```python
from build123d import *

# Parameters (mm, degrees)
BOSS_EXTRU_1_DEPTH      = 3
ESQUISSE2_R             = 1.25
ENL_V_MAT_EXTRU_1_DEPTH = 8
ESQUISSE3_W             = 6
ESQUISSE3_H             = 5
BOSS_EXTRU_2_DEPTH      = 5
ENL_V_MAT_EXTRU_3_DEPTH = 7
CONG_4_R                = 0.5
CONG_5_R                = 1
ENL_V_MAT_EXTRU_5_DEPTH = 7


with BuildPart() as part:
    # Esquisse1 → Boss.-Extru.1 (new body, symmetric)
    with BuildSketch(Plane.XY):
        Polygon((-6, 0), (-2.4, 0), (-2.4, -2), (2.4, -2), (2.4, 0), (6, 0), (6, 5), (-6, 5), align=None)
    extrude(amount=BOSS_EXTRU_1_DEPTH, both=True)

    # Esquisse2 → Enlèv. mat.-Extru.1 (cut, through all)
    with BuildSketch(Plane(origin=(0, 5, 0), x_dir=(1, 0, 0), z_dir=(0, 1, 0))):
        Circle(ESQUISSE2_R)
    extrude(amount=-ENL_V_MAT_EXTRU_1_DEPTH, mode=Mode.SUBTRACT)

    # Esquisse3 → Boss.-Extru.2 (add)
    with BuildSketch(Plane.ZY.offset(6)):
        with Locations((0, 2.5)):
            Rectangle(ESQUISSE3_W, ESQUISSE3_H)
    extrude(amount=BOSS_EXTRU_2_DEPTH)

    # Esquisse7 → Enlèv. mat.-Extru.3 (cut, through all)
    with BuildSketch(Plane.XY.offset(3)):
        Polygon((-11, 5), (-9.556624327, 2.5), (-11, 0), align=None)
    extrude(amount=-ENL_V_MAT_EXTRU_3_DEPTH, mode=Mode.SUBTRACT)

    # Congé4
    cong_4_edges = [part.edges().sort_by_distance(p)[0] for p in [
        (6, 0, 0),
        (2.4, -2, 0),
        (-2.4, -2, 0),
        (6, 5, 0),
        (-11, 0, 0),
        (-11, 5, 0),
    ]]
    fillet(cong_4_edges, radius=CONG_4_R)

    # Congé5
    cong_5_edges = [part.edges().sort_by_distance(p)[0] for p in [
        (-9.556624327, 2.5, 0),
    ]]
    fillet(cong_5_edges, radius=CONG_5_R)

    # Esquisse12 → Enlèv. mat.-Extru.5 (cut, through all)
    with BuildSketch(Plane(origin=(0, 0, -3), x_dir=(-1, 0, 0), z_dir=(0, 0, -1))):
        with BuildLine():
            Line((-4.279385242, 0), (-2.4, -0.684040287))
            ThreePointArc((-2.4, -0.684040287), (-2.997672477, 0.597672477), (-4.279385242, 0))
        make_face()
        with BuildLine():
            Line((4.279385242, 0), (2.4, -0.684040287))
            ThreePointArc((2.4, -0.684040287), (2.997672477, 0.597672477), (4.279385242, 0))
        make_face()
    extrude(amount=-ENL_V_MAT_EXTRU_5_DEPTH, mode=Mode.SUBTRACT)


solid = part.part
```
The listing builds one solid part. Answer for the finished solid, in the listing's coordinates (mm). A direction names the side the tool comes from. Coordinates: 2 decimals unless noted, no trailing zeros. Loops run counter-clockwise (first coordinate to the right, second up) from the corner with the lowest first, then second, coordinate; pieces in that order, holes last. Notation, with made-up numbers: (68, 61) - (123, 61) arc R9 cw to (123, 70) - close; hole circle Ø7 at (68.5, 83). An arc over 180 degrees is marked (long way). Write item = value, one per line.
1) Section B-B (x = 0) is taken. Determine the outline of the cut face in (y, z), plus the area to 3 significant figures.
Responses:
outline = (-2, -3) - (5, -3) - (5, -1.25) - (-2, -1.25) - close; (-2, 1.25) - (5, 1.25) - (5, 3) - (-2, 3) - close
area = 24.5 mm^2
2) Each of these flat-tipped pins is pushed along its axis until it touches: P1, Ø0.9, axis at y = -1, z = -1, coming from the -X side; P2, Ø0.9, axis at y = -1, z = -1.5, coming from the +X side; P3, Ø3, axis at x = -3.5, z = -1, coming from the -Y side. Where does it stop, or does it pass through?
Responses:
P1 = -2.4
P2 = 2.4
P3 = -1.99
3) Find the intervals of material crossed by line 1 along X through (y, z) = (0.5, 0.5); line 2 along X through (y, z) = (1.5, 0); line 3 along Z through (x, y) = (0, 2), in increasing order.
Responses:
line_1 = -10.63 to -3.88, -2.8 to -1.15, 1.15 to 2.8, 3.88 to 6
line_2 = -10.13 to -1.25, 1.25 to 6
line_3 = -3 to -1.25, 1.25 to 3
4) Section C-C (y = 1.5) is taken. Determine the outline of the cut face in (x, z), plus the area to 3 significant figures.
Responses:
outline = (-10.13, -3) - (6, -3) - (6, 3) - (-10.13, 3) - close; hole circle Ø2.5 at (0, 0)
area = 91.9 mm^2
5) Section D-D (z = -1.75) is taken. Determine the outline of the cut face in (x, y).
Responses:
outline = (-10.57, 0.75) arc R0.5 ccw to (-10.13, 0) - (-4.28, 0) arc R1 cw to (-2.4, -0.68) - (-2.4, -1.5) arc R0.5 ccw to (-1.9, -2) - (1.9, -2) arc R0.5 ccw to (2.4, -1.5) - (2.4, -0.68) arc R1 cw to (4.28, 0) - (5.5, 0) arc R0.5 ccw to (6, 0.5) - (6, 4.5) arc R0.5 ccw to (5.5, 5) - (-10.13, 5) arc R0.5 ccw to (-10.57, 4.25) - (-9.85, 3) arc R1 cw to (-9.85, 2) - close
6) Which of the six approach directions +Z, -Z, +X, -X, +Y, -Y give full straight-line access (tool end or side, diameter ignored) to faces 4 (the face through (-2.4, -1, 0)), 5 (the face through (5, 0, 0)), 6 (the face through (-10.21, 3.63, 0.04))?
Responses:
face_4 = +Z, -Z, -X, -Y
face_5 = +Z, -Z, +X, -Y
face_6 = +Z, -Z, -X
7) Determine the mould class of faces 1 (the face through (-7, 0, 0)), 2 (the face through (-10.201, 1.384, 0.042)), 3 (the face through (2.4, -1, 0)) for opening direction Y: pulls with the +Y half, pulls with the -Y half, needs draft (parallel to the pull), parting line crosses it, or undercut.
Responses:
face_1 = pulls with the -Y half
face_2 = undercut
face_3 = needs draft
8) Section A-A (z = 0) is taken. Determine the outline of the cut face in (x, y).
Responses:
outline = (-10.57, 0.75) arc R0.5 ccw to (-10.13, 0) - (-4.28, 0) arc R1 cw to (-2.4, -0.68) - (-2.4, -1.5) arc R0.5 ccw to (-1.9, -2) - (-1.25, -2) - (-1.25, 5) - (-10.13, 5) arc R0.5 ccw to (-10.57, 4.25) - (-9.85, 3) arc R1 cw to (-9.85, 2) - close; (1.25, -2) - (1.9, -2) arc R0.5 ccw to (2.4, -1.5) - (2.4, -0.68) arc R1 cw to (4.28, 0) - (5.5, 0) arc R0.5 ccw to (6, 0.5) - (6, 4.5) arc R0.5 ccw to (5.5, 5) - (1.25, 5) - close
